from build123d import *

# Parameters (mm, degrees)
SKETCH1_R           = 5.5
BOSS_EXTRUDE1_DEPTH = 5
SKETCH3_R           = 4.2
BOSS_EXTRUDE3_DEPTH = 5
BOSS_EXTRUDE2_DEPTH = 69


with BuildPart() as part:
    # Sketch1 → Boss-Extrude1 (new body)
    with BuildSketch(Plane(origin=(0, 0, 0), x_dir=(0, 1, 0), z_dir=(0, 0, 1))):
        with Locations(Location((0, 0, 0), (0, 0, 270))):
            Circle(SKETCH1_R)
    extrude(amount=BOSS_EXTRUDE1_DEPTH)

    # Sketch3 → Boss-Extrude3 (add)
    with BuildSketch(Plane.XY.offset(5)):
        Circle(SKETCH3_R)
    extrude(amount=BOSS_EXTRUDE3_DEPTH)

    # Sketch2 → Boss-Extrude2 (add)
    with BuildSketch(Plane.XY.offset(10)):
        with BuildLine():
            Line((-0.834166667, 3.775921626), (0.965833333, 3.775921626))
            Line((0.965833333, 3.775921626), (0.965833333, 2.775921626))
            ThreePointArc((0.965833333, 2.775921626), (-0.13585463, -2.948190479), (-0.834166667, 2.838996753))
            Line((-0.834166667, 2.838996753), (-0.834166667, 3.775921626))
        make_face()
    extrude(amount=BOSS_EXTRUDE2_DEPTH)


solid = part.part
Part model, mm, in its own coordinate system. A direction names the side the tool comes from. Coordinates: 2 decimals unless noted, no trailing zeros. Order: outer loops, then holes, each group sorted by start corner. A loop starts at its lowest first (then second) coordinate and runs counter-clockwise, first axis right, second up. Notation, with made-up numbers: M 29,46 L 81,46 A26 ccw 81,74 Z; hole C 83,72.5 d7. An arc over 180 degrees is marked long. Use a Markdown table: item, result.
(1) Cut at A-A on y = 0. Write the cut outline in (x, z), then the cut area to 3 significant figures.
A:
| item | result |
|---|---|
| outline | M -5.5,0 L 5.5,0 L 5.5,5 L 4.2,5 L 4.2,10 L 2.92,10 L 2.92,79 L -2.98,79 L -2.98,10 L -4.2,10 L -4.2,5 L -5.5,5 Z |
| area | 504 mm^2 |
(2) Probe L1, parallel to Z at x = -2.75, y = -2.75; L2, parallel to Z at x = 1, y = 5; L3, parallel to Y at x = 0, z = 47. List the from-to ranges inside material, lowest first.
A:
| item | result |
|---|---|
| L1 | z = 0 to 10 |
| L2 | z = 0 to 5 |
| L3 | y = -2.95 to 3.78 |
(3) Tool access for faces 1 (the cylindrical face through (-0.02, -2.95, 44.02)), 2 (the flat face through (0, 0, 79)), 3 (the flat face through (0, 3.776, 44)): list every direction of +Z, -Z, +X, -X, +Y, -Y with a clear straight run to the whole face (end or side of a thin tool).
A:
| item | result |
|---|---|
| face 1 | +Z |
| face 2 | +Z, +X, -X, +Y, -Y |
| face 3 | +Z, +X, -X, +Y |
(4) Flat gauge pins, fed straight in: pin 1 (3 mm diameter, centred on x = 1, z = 51, fed in from -Y); pin 2 (3.5 mm diameter, centred on x = -2, y = -2.5, fed in from +Z); pin 3 (1.5 mm diameter, centred on x = -2, z = 39, fed in from +Y); pin 4 (2 mm diameter, centred on y = -1, z = 26, fed in from +X). Where does each tip first touch, or does it go through?
A:
| item | result |
|---|---|
| pin 1 | stops at y = -2.95 |
| pin 2 | stops at z = 79 |
| pin 3 | stops at y = 2.69 |
| pin 4 | stops at x = 2.92 |
(5) Cut at C-C on z = 72.5. Write the cut outline in (x, y).
A:
| item | result |
|---|---|
| outline | M -0.83,2.84 A2.95 ccw long 0.97,2.78 L 0.97,3.78 L -0.83,3.78 Z |
(6) Cut at B-B on x = 0. Write the cut outline in (y, z).
A:
| item | result |
|---|---|
| outline | M -5.5,0 L 5.5,0 L 5.5,5 L 4.2,5 L 4.2,10 L 3.78,10 L 3.78,79 L -2.95,79 L -2.95,10 L -4.2,10 L -4.2,5 L -5.5,5 Z |
